Build history of the part. All positions in model axes, mm. A direction names the side the tool comes from. Coordinates: 2 decimals unless noted, no trailing zeros. Write each loop counter-clockwise with the first axis right and the second up, starting at its lowest first coordinate (ties: lowest second). Pieces come first, ordered by that corner, then holes.
from build123d import *

# Parameters (mm, degrees)
F0_R     = 1
F1_DEPTH = 5


with BuildPart() as f1:
    # F0 (on Top) → F1 (new body)
    with BuildSketch(Plane.XY):
        with BuildLine():
            Line((25.1, 0), (0.5, 0))
            ThreePointArc((0.5, 0), (0.146447, -0.146447), (0, -0.5))
            Line((0, -0.5), (0, -9.5))
            ThreePointArc((0, -9.5), (0.146447, -9.853553), (0.5, -10))
            Line((0.5, -10), (25.1, -10))
            Line((25.1, -10), (25.1, -9.999452))
            ThreePointArc((25.1, -9.999452), (24.367767, -8.231685), (22.6, -7.499452))
            Line((22.6, -7.499452), (21.152357, -7.499452))
            ThreePointArc((21.152357, -7.499452), (18.603039, -5.123229), (20.905998, -2.507539))
            ThreePointArc((20.905998, -2.507539), (21.1, -2.5), (21.294002, -2.507539))
            Line((21.294002, -2.507539), (22.6, -2.507539))
            ThreePointArc((22.6, -2.507539), (24.367767, -1.775306), (25.1, -0.007539))
            Line((25.1, -0.007539), (25.1, 0))
        make_face()
        with Locations((14, -5)):
            Circle(F0_R, mode=Mode.SUBTRACT)
    extrude(amount=F1_DEPTH)


solid = f1.part
(1) Slice it at D-D, the plane y = -3.5. List the corners of the cut face in (x, z).
(2) 3-axis set-ups, long thin cutter, end or side, ignore diameter. For faces 1 (the flat face through (13, 0, 2)), 2 (the flat face through (22, -7.499, 2)): which of +Z, -Z, +X, -X, +Y, -Y reach the whole face in a straight line?
(3) Two-plate mould, pull along Y, no slides. Class faces 3 (the cylindrical face through (24.348, -1.795, 2.465)), 4 (the flat face through (13, -10, 2)), 5 (the flat face through (12, -5, 0)), 6 (the cylindrical face through (24.387, -8.251, 2.465)): pulls with the +Y half, pulls with the -Y half, needs draft (parallel to the pull), parting line crosses it, or undercut.
(4) Probe L1, parallel to Y at x = 14, z = 4.05; L2, parallel to X at y = -5.25, z = 3.7; L3, parallel to Y at x = 20.5, z = 2.45. List the from-to ranges inside material, lowest first.
(5) Slice it at A-A, the plane x = 14. List the corners of the cut face in (y, z).
(6) Slice it at B-B, the plane y = -5. List the corners of the cut face in (x, z), and give its area (3 significant figures).
Results:
1. outline: (0, 0) - (19.1, 0) - (19.1, 5) - (0, 5) - close
2. face 1: +Z, -Z, +X, -X, +Y
2. face 2: +Z, -Z, +X
3. face 3: undercut
3. face 4: pulls with the -Y half
3. face 5: needs draft
3. face 6: undercut
4. L1: y = -10 to -6, -4 to 0
4. L2: x = 0 to 13.03, 14.97 to 18.61
4. L3: y = -10 to -7.43, -2.57 to 0
5. outline: (-10, 0) - (-6, 0) - (-6, 5) - (-10, 5) - close; (-4, 0) - (0, 0) - (0, 5) - (-4, 5) - close
6. outline: (0, 0) - (13, 0) - (13, 5) - (0, 5) - close; (15, 0) - (18.6, 0) - (18.6, 5) - (15, 5) - close
6. area: 83.0 mm2
